The model under review builds one solid part; all positions refer to its coordinate system, in mm. Face numbers are marked on the shaded views. A direction names the side the tool comes from. Coordinates: 2 decimals unless noted, no trailing zeros. Order: outer loops, then holes, each group sorted by start corner. A loop starts at its lowest first (then second) coordinate and runs counter-clockwise, first axis right, second up. Notation, with made-up numbers: M 76,9 L 90,9 A12 ccw 90,15 Z; hole C 61.5,-8 d5. An arc over 180 degrees is marked long. Answer as CSV lines item,"result". Start each with the question number.
Q1. Consider section A-A on x = 196. Write out the cut boundary in (y, z) (3 decimals).
Q2. Consider section C-C on y = -51. Write out the cut boundary in (x, z) (3 decimals).
Q3. For P1, Ø3, axis at y = 18.5, z = -104, coming from the +X side; P2, Ø3, axis at y = 15.5, z = -103, coming from the -X side; P3, Ø0.9, axis at x = 359, y = -1.5, coming from the -Z side, all flat-tipped, find the tip position at first contact; note any pin that passes through.
Q4. Wall thickness on L1, parallel to Z at x = 149.5, y = 2.5; L2, parallel to Y at x = -117, z = 26; L3, parallel to X at y = -2.5, z = -62.5: over which ranges is each line inside the solid? List them lowest first. Write a range as [from, to].
Q5. Consider section B-B on z = 16. Write out the cut boundary in (x, y).
Q6. Machinability: for the marked faces 1, 2 and 3, which of the approach directions +Z, -Z, +X, -X, +Y, -Y give a long, thin tool a straight path to every point of the face, cutting with its end or side? Answer none if there is none.
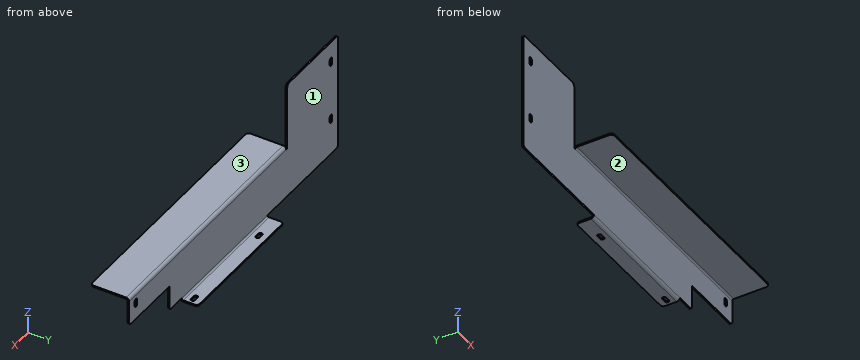
from build123d import *

# Parameters (mm, degrees)
BASE_FLANGE1_DEPTH       = 3.03784
EDGE_FLANGE1_DEPTH       = 278
EDGE_FLANGE2_DEPTH       = 508.825
M6_START                 = -106.21284
M6_CLEARANCE_SLOT1_DEPTH = 3.03784
M6_START_2               = -3.03784
M6_CLEARANCE_SLOT2_DEPTH = 3.03784
FILLET1_R                = 6


# Read off the part's stored shape, not the designer's step: M6 Clearance Slot1, M6 Clearance Slot2
# Sheet-metal steps are written as plain solids
with BuildPart() as part:
    # Sketch1 → Base-Flange1 (new body)
    with BuildSketch(Plane(origin=(0, 0, 0), x_dir=(1, 0, 0), z_dir=(0, 1, 0))):
        Polygon((0, -135), (0, 0), (512, 0), (512, 50), (382, 50), (382, 100), (-165, 100), (-165, -135), align=None)
    extrude(amount=-BASE_FLANGE1_DEPTH)

    # Edge-Flange1 section (across the edge) → Edge-Flange1 (add)
    with BuildSketch(Plane(origin=(342, 0, -103.175), x_dir=(0, 0, 1), z_dir=(-1, 0, 0))):
        with BuildLine():
            Line((-3.03784, 3.175), (-3.03784, 32))
            Line((-3.03784, 32), (0, 32))
            Line((0, 32), (0, 3.175))
            ThreePointArc((0, 3.175), (0.92993597, 0.92993597), (3.175, 0))
            Line((3.175, 0), (3.175, -3.03784))
            ThreePointArc((3.175, -3.03784), (-1.218141294, -1.218141294), (-3.03784, 3.175))
        make_face()
    extrude(amount=EDGE_FLANGE1_DEPTH)

    # Edge-Flange2 section (across the edge) → Edge-Flange2 (add)
    with BuildSketch(Plane(origin=(512, -3.03784, 3.175), x_dir=(0, 0, -1), z_dir=(-1, 0, 0))):
        with BuildLine():
            Line((-3.03784, 3.175), (-3.03784, 74))
            Line((-3.03784, 74), (0, 74))
            Line((0, 74), (0, 3.175))
            ThreePointArc((0, 3.175), (0.92993597, 0.92993597), (3.175, 0))
            Line((3.175, 0), (3.175, -3.03784))
            ThreePointArc((3.175, -3.03784), (-1.218141294, -1.218141294), (-3.03784, 3.175))
        make_face()
    extrude(amount=EDGE_FLANGE2_DEPTH)

    # M6 Clearance Slot1 outline → M6 Clearance Slot1 (cut)
    with BuildSketch(Plane.XY.offset(M6_START)):
        with BuildLine():
            Line((112.7, 12), (121.3, 12))
            ThreePointArc((121.3, 12), (125.3, 16), (121.3, 20))
            Line((121.3, 20), (112.7, 20))
            ThreePointArc((112.7, 20), (108.7, 16), (112.7, 12))
        make_face()
        with BuildLine():
            ThreePointArc((331.3, 12), (335.3, 16), (331.3, 20))
            Line((331.3, 20), (322.7, 20))
            ThreePointArc((322.7, 20), (318.7, 16), (322.7, 12))
            Line((322.7, 12), (331.3, 12))
        make_face()
    extrude(amount=M6_CLEARANCE_SLOT1_DEPTH, mode=Mode.SUBTRACT)

    # M6 Clearance Slot2 outline → M6 Clearance Slot2 (cut)
    with BuildSketch(Plane(origin=(0, 0, 0), x_dir=(1, 0, 0), z_dir=(0, 1, 0)).offset(M6_START_2)):
        with BuildLine():
            Line((-137.57432, -98.08716), (-137.57432, -89.48716))
            ThreePointArc((-137.57432, -89.48716), (-141.57432, -85.48716), (-145.57432, -89.48716))
            Line((-145.57432, -89.48716), (-145.57432, -98.08716))
            ThreePointArc((-145.57432, -98.08716), (-141.57432, -102.08716), (-137.57432, -98.08716))
        make_face()
        with BuildLine():
            ThreePointArc((-137.57432, 30.51284), (-141.57432, 34.51284), (-145.57432, 30.51284))
            Line((-145.57432, 30.51284), (-145.57432, 21.91284))
            ThreePointArc((-145.57432, 21.91284), (-141.57432, 17.91284), (-137.57432, 21.91284))
            Line((-137.57432, 21.91284), (-137.57432, 30.51284))
        make_face()
        with BuildLine():
            Line((494.42568, 11.91284), (494.42568, 20.51284))
            ThreePointArc((494.42568, 20.51284), (490.42568, 24.51284), (486.42568, 20.51284))
            Line((486.42568, 20.51284), (486.42568, 11.91284))
            ThreePointArc((486.42568, 11.91284), (490.42568, 7.91284), (494.42568, 11.91284))
        make_face()
    extrude(amount=M6_CLEARANCE_SLOT2_DEPTH, mode=Mode.SUBTRACT)

    # Fillet1
    fillet1_edges = [part.edges().sort_by_distance(p)[0] for p in [
        (-165, -1.51892, -100),
        (382, -1.51892, -100),
        (512, -1.51892, -50),
        (0, -1.51892, 135),
        (-165, -1.51892, 135),
        (342, 32, -104.69392),
        (64, 32, -104.69392),
        (512, -77.03784, 4.69392),
        (3.175, -77.03784, 4.69392),
    ]]
    fillet(fillet1_edges, radius=FILLET1_R)


solid = part.part
Evaluation:
1,outline,"M -77.038,3.175 L -6.213,3.175 A3.175 cw -3.038,0 L -3.038,-100 A6.213 ccw 3.175,-106.213 L 32,-106.213 L 32,-103.175 L 3.175,-103.175 A3.175 cw 0,-100 L 0,0 A6.213 ccw -6.213,6.213 L -77.038,6.213 Z"
2,outline,"M 3.175,3.175 L 512,3.175 L 512,6.213 L 3.175,6.213 Z"
3,P1,"stops at x = 342"
3,P2,"stops at x = 64"
3,P3,"stops at z = -100"
4,L1,"z = [-106.18, -103.1]"
4,L2,"y = [-3.04, 0]"
4,L3,"x = [-165, 382]"
5,outline,"M -165,-3.04 L 0,-3.04 L 0,0 L -165,0 Z"
6,face 1,"+Z, +X, -X, +Y"
6,face 2,"-Z, +X, -X, -Y"
6,face 3,"+Z, +X, -X, +Y, -Y"
